Job drawing, mm, ordinate dimensions from the low corner. One solid piece. A direction names the side the tool comes from. Give positions to 0.01 mm unless a question says otherwise; leave off trailing zeros. Write each loop counter-clockwise with the first axis right and the second up, starting at its lowest first coordinate (ties: lowest second). Pieces come first, ordered by that corner, then holes. Notation, with made-up numbers: (-12, 50.25) -> (34, 50.25) arc R19 cw to (34, 56.25) -> close; hole circle Ø1 at (74.5, -7). An arc over 180 degrees is marked (long way). One line per question, with ' | ' between items. Start each with the question number.
(1) Drill centre lines: probe 1 along Y at (x, z) = (4, 18.5); probe 2 along X at (y, z) = (3, 12.5); probe 3 along Z at (x, y) = (8, 1.25). Where is each one in solid material? Low to high. Write a range as from..to.
(2) Band-saw the part on B-B, the plane x = 12.7. Give the cut face in (y, z) (3 decimals).
(3) Band-saw the part on C-C, the plane y = 5.5. Give the cut face in (x, z) (3 decimals), and give its area (3 significant figures).
(4) Tool access for the marked faces 1, 2 and 3: list every direction of +Z, -Z, +X, -X, +Y, -Y with a clear straight run to the whole face (end or side of a thin tool).
(5) Band-saw the part on A-A, the plane z = 12.7. Give the cut face in (x, y) (3 decimals), and give its area (3 significant figures).
(6) Band-saw the part on D-D, the plane z = 4.25. Give the cut face in (x, y).
(7) Pin check, flat tips, straight feed: P1, Ø6, axis at x = 11, z = 2.5, coming from the -Y side; P2, Ø4, axis at x = 9.5, y = 11, coming from the +Z side; P3, Ø5, axis at x = 10.5, y = 8, coming from the -Z side; P4, Ø4, axis at y = 3.5, z = 3, coming from the -X side. Stop position of each tip, or through.
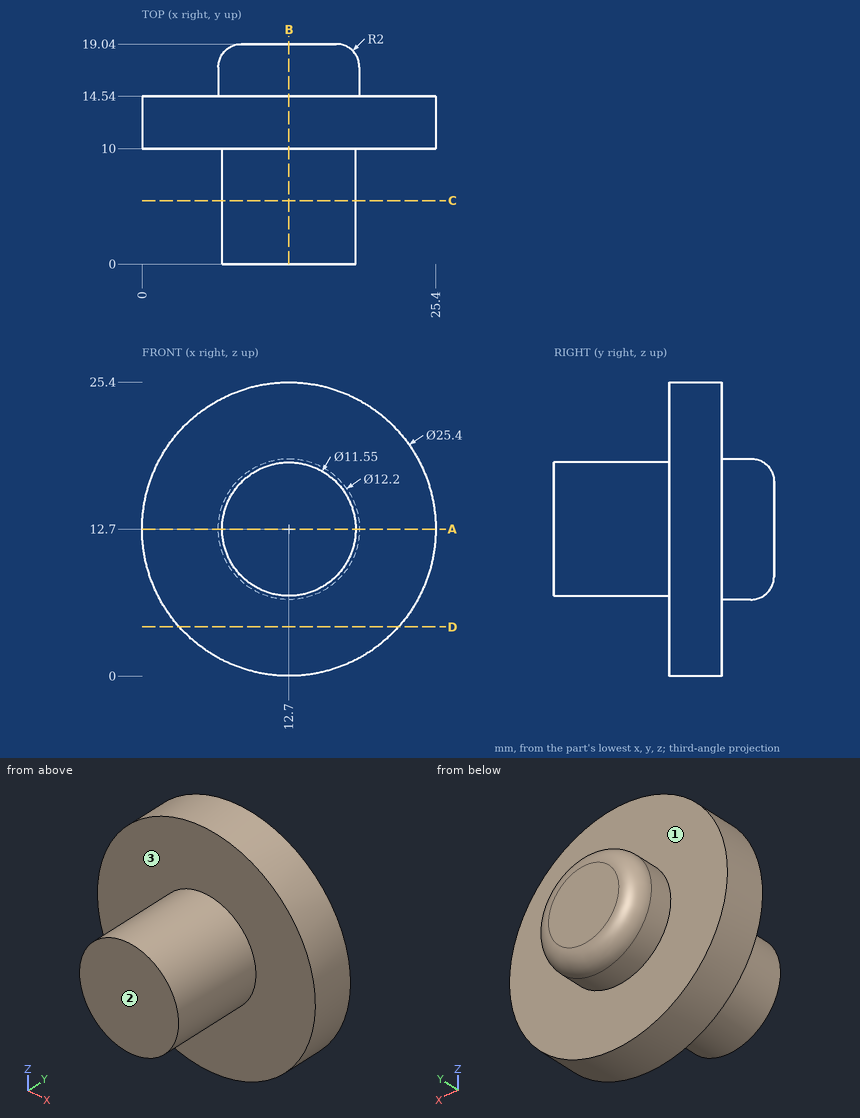
Results:
1) probe 1: y = 10..14.54 | probe 2: x = 6.93..18.47 | probe 3: z = 9.34..16.06
2) outline: (0, 6.925) -> (10, 6.925) -> (10, 0) -> (14.54, 0) -> (14.54, 6.6) -> (17.04, 6.6) arc R2 ccw to (19.04, 8.6) -> (19.04, 16.8) arc R2 ccw to (17.04, 18.8) -> (14.54, 18.8) -> (14.54, 25.4) -> (10, 25.4) -> (10, 18.475) -> (0, 18.475) -> close
3) outline: circle Ø11.55 at (12.7, 12.7) | area: 105 mm²
4) face 1: +Y | face 2: +Z, -Z, +X, -X, -Y | face 3: -Y
5) outline: (0, 10) -> (6.925, 10) -> (6.925, 0) -> (18.475, 0) -> (18.475, 10) -> (25.4, 10) -> (25.4, 14.54) -> (18.8, 14.54) -> (18.8, 17.04) arc R2 ccw to (16.8, 19.04) -> (8.6, 19.04) arc R2 ccw to (6.6, 17.04) -> (6.6, 14.54) -> (0, 14.54) -> close | area: 284 mm²
6) outline: (3.22, 10) -> (22.18, 10) -> (22.18, 14.54) -> (3.22, 14.54) -> close
7) P1: stops at y = 10 | P2: stops at z = 25.34 | P3: stops at z = 0.02 | P4: passes through
